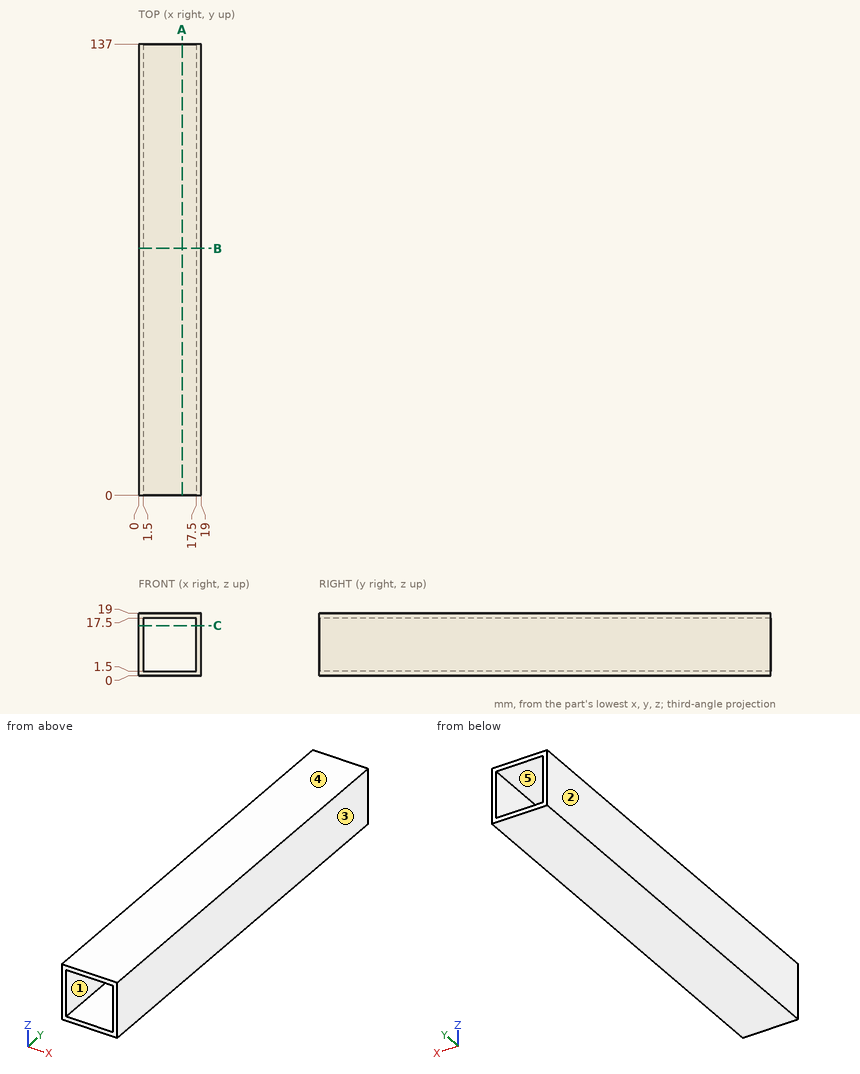
Geometry: see drawing. Coordinates: mm, zero at the bounding-box minimum. A direction names the side the tool comes from. Round coordinates to 2 decimals unless told otherwise and drop trailing zeros. Loops run counter-clockwise (first coordinate to the right, second up) from the corner with the lowest first, then second, coordinate; pieces in that order, holes last. Notation, with made-up numbers: (-3, -36.5) -> (43, -36.5) arc R17 ccw to (43, -22.5) -> close; hole circle Ø11 at (79.25, 55). An arc over 180 degrees is marked (long way). One line per question, with ' | ' between items. Start each with the question number.
1. Set-up query: the marked faces 4 and 5. Return all of +Z, -Z, +X, -X, +Y, -Y with unobstructed straight access to the full face (end or side cutting, diameter ignored); none if empty.
2. Section B-B on y = 75. Output: boundary loops of the cut face in (x, z), and give its area (3 significant figures).
3. Mould query, pull axis X, two halves, no side actions, for the marked faces 1, 2 and 3. Classes: pulls with the +X half, pulls with the -X half, needs draft (parallel to the pull), parting line crosses it, or undercut.
4. Line query: line 1 along X through (y, z) = (90, 13.75). Output: solid intervals per line, ascending. Write a range as [from, to].
5. Section C-C on z = 15.25. Output: boundary loops of the cut face in (x, y).
6. Section A-A on x = 13.25. Output: boundary loops of the cut face in (y, z), and give its area (3 significant figures).
Returned:
1) face 4: +Z, +X, -X, +Y, -Y | face 5: +Y, -Y
2) outline: (0, 0) -> (19, 0) -> (19, 19) -> (0, 19) -> close; hole (1.5, 1.5) -> (17.5, 1.5) -> (17.5, 17.5) -> (1.5, 17.5) -> close | area: 105 mm2
3) face 1: undercut | face 2: pulls with the -X half | face 3: pulls with the +X half
4) line 1: x = [0, 1.5], [17.5, 19]
5) outline: (0, 0) -> (1.5, 0) -> (1.5, 137) -> (0, 137) -> close; (17.5, 0) -> (19, 0) -> (19, 137) -> (17.5, 137) -> close
6) outline: (0, 0) -> (137, 0) -> (137, 1.5) -> (0, 1.5) -> close; (0, 17.5) -> (137, 17.5) -> (137, 19) -> (0, 19) -> close | area: 411 mm2
